Geometry check sheet. Reference: the model listing, model coordinates, mm. Give positions to 0.01 mm unless a question says otherwise; leave off trailing zeros. Order: outer loops, then holes, each group sorted by start corner. A loop starts at its lowest first (then second) coordinate and runs counter-clockwise, first axis right, second up.
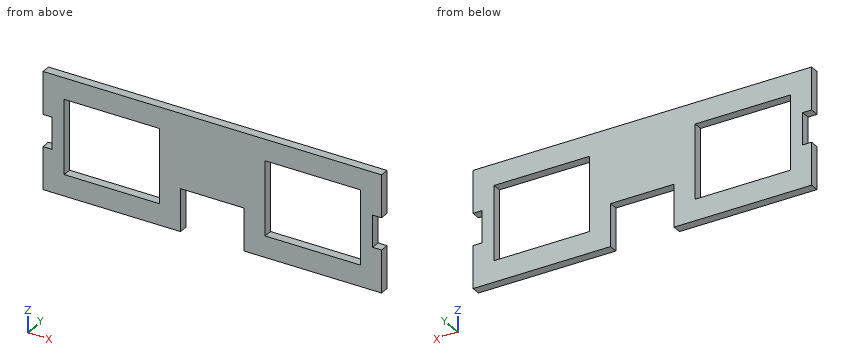
```python
from build123d import *

# Parameters (mm, degrees)
SKETCH1_W              = 203.2
SKETCH1_H              = 69.85
BASE_DEPTH             = 5.334
SKETCH2_W              = 5.334
SKETCH2_H              = 19.05
SLOTS_DEPTH            = 215.936534949
SKETCH3_W              = 38.1
SKETCH3_H              = 25.4
CENTER_CUTOUT_DEPTH    = 215.936534949
WEIGHT_REDUCTION_DEPTH = 215.936534949


with BuildPart() as part:
    # Sketch1 → Base (new body)
    with BuildSketch(Plane(origin=(0, 0, 0), x_dir=(1, 0, 0), z_dir=(0, 1, 0))):
        with Locations((101.6, 34.925)):
            Rectangle(SKETCH1_W, SKETCH1_H)
    extrude(amount=BASE_DEPTH)

    # Sketch2 → Slots (cut, through all)
    with BuildSketch(Plane(origin=(0, 5.334, 0), x_dir=(1, 0, 0), z_dir=(0, 1, 0))):
        with Locations((2.667, 34.925)):
            Rectangle(SKETCH2_W, SKETCH2_H)
        with Locations((200.533, 34.925)):
            Rectangle(SKETCH2_W, SKETCH2_H)
    extrude(amount=-SLOTS_DEPTH, mode=Mode.SUBTRACT)

    # Sketch3 → Center Cutout (cut, through all)
    with BuildSketch(Plane(origin=(0, 5.334, 0), x_dir=(1, 0, 0), z_dir=(0, 1, 0))):
        with Locations((101.6, 57.15)):
            Rectangle(SKETCH3_W, SKETCH3_H)
    extrude(amount=-CENTER_CUTOUT_DEPTH, mode=Mode.SUBTRACT)

    # Sketch4 → Weight Reduction (cut, through all)
    with BuildSketch(Plane(origin=(0, 5.334, 0), x_dir=(1, 0, 0), z_dir=(0, 1, 0))):
        Polygon((69.85, 44.45), (69.85, 57.15), (12.7, 57.15), (12.7, 44.45), (12.7, 25.4), (12.7, 12.7), (69.85, 12.7), align=None)
        Polygon((190.5, 25.4), (190.5, 12.7), (133.35, 12.7), (133.35, 44.45), (133.35, 57.15), (190.5, 57.15), (190.5, 44.45), align=None)
    extrude(amount=-WEIGHT_REDUCTION_DEPTH, mode=Mode.SUBTRACT)


solid = part.part
```
Q1. Cross-section at B-B, the plane x = 138. Record the boundary of the cut face in (y, z).
Q2. Cross-section at D-D, the plane y = 2.5. Record the boundary of the cut face in (x, z).
Q3. Gauge pin test, flat ends, axial feed: P1, Ø1.6, axis at x = 105.5, y = 2.5, coming from the -Z side; P2, Ø2.5, axis at y = 2.5, z = -38.5, coming from the +X side; P3, Ø2.5, axis at y = 2.5, z = -28, coming from the -X side. Record the tip position at first contact, or that the pin passes through.
Q4. Thickness scan on L1, parallel to X at y = 0.6, z = -21.5; L2, parallel to X at y = 2.05, z = -45.5; L3, parallel to X at y = 2.8, z = -29. Record the ranges inside material, lowest first.
Q5. Cross-section at C-C, the plane z = -28.5. Record the boundary of the cut face in (x, y).
Q6. Cross-section at A-A, the plane z = -47.5. Record the boundary of the cut face in (x, y).
Answers follow:
1. outline: (0, -69.85) - (5.33, -69.85) - (5.33, -57.15) - (0, -57.15) - close; (0, -12.7) - (5.33, -12.7) - (5.33, 0) - (0, 0) - close
2. outline: (0, -69.85) - (82.55, -69.85) - (82.55, -44.45) - (120.65, -44.45) - (120.65, -69.85) - (203.2, -69.85) - (203.2, -44.45) - (197.87, -44.45) - (197.87, -25.4) - (203.2, -25.4) - (203.2, 0) - (0, 0) - (0, -25.4) - (5.33, -25.4) - (5.33, -44.45) - (0, -44.45) - close; hole (12.7, -57.15) - (69.85, -57.15) - (69.85, -12.7) - (12.7, -12.7) - close; hole (133.35, -57.15) - (190.5, -57.15) - (190.5, -12.7) - (133.35, -12.7) - close
3. P1: stops at z = -44.45
3. P2: stops at x = 197.87
3. P3: stops at x = 5.33
4. L1: x = 0 to 12.7, 69.85 to 133.35, 190.5 to 203.2
4. L2: x = 0 to 12.7, 69.85 to 82.55, 120.65 to 133.35, 190.5 to 203.2
4. L3: x = 5.33 to 12.7, 69.85 to 133.35, 190.5 to 197.87
5. outline: (5.33, 0) - (12.7, 0) - (12.7, 5.33) - (5.33, 5.33) - close; (69.85, 0) - (133.35, 0) - (133.35, 5.33) - (69.85, 5.33) - close; (190.5, 0) - (197.87, 0) - (197.87, 5.33) - (190.5, 5.33) - close
6. outline: (0, 0) - (12.7, 0) - (12.7, 5.33) - (0, 5.33) - close; (69.85, 0) - (82.55, 0) - (82.55, 5.33) - (69.85, 5.33) - close; (120.65, 0) - (133.35, 0) - (133.35, 5.33) - (120.65, 5.33) - close; (190.5, 0) - (203.2, 0) - (203.2, 5.33) - (190.5, 5.33) - close
